Autodesk Inventor part; units mm, degrees
ref_plane "YZ Plane" through (0, 0, 0) normal (1, 0, 0) x (0, 1, 0)
ref_plane "XZ Plane" through (0, 0, 0) normal (0, 1, 0) x (-1, 0, 0)
ref_plane "XY Plane" through (0, 0, 0) normal (0, 0, 1) x (1, 0, 0)
sketch "Sketch1" plane through (0, 0, 0) normal (0, 0, 1) x (1, 0, 0)
  circle A0 centre (0, 0) radius 55
  arc A1 (-1.4, -192.7776) -> (1.4, -192.7776) centre (0, -192.7776) ccw
  line L0 (-95, 160) -> (105, 160)
  line L1 (105, 160) -> (105, -240)
  line L2 (105, -240) -> (-95, -240)
  line L3 (-95, -240) -> (-95, 160)
  line L4 (-95, 200) -> (95, -200) construction
  line L5 (95, 200) -> (-95, -200) construction
  line L6 (0, 0) -> (0, -40) construction
  point P0 (0, 0)
  dimension "d58" = 200
  dimension "d59" = 400
  dimension "d60" = 40
extrude "Extrusion1" add sketch "Sketch1" against normal blind 5
sketch "Sketch2" plane through (0, 0, 0) normal (0, 0, 1) x (1, 0, 0)
  circle A0 centre (-22.5, -100.6741) radius 2.25
  circle A1 centre (22.5, -100.6741) radius 2.25
  circle A2 centre (22.5, -71.1776) radius 2
  circle A3 centre (-22.5, -71.1776) radius 2
  circle A4 centre (-22.5, -162.7577) radius 2.25
  circle A5 centre (22.5, -162.7577) radius 2.25
  point P0 (0, 0)
  dimension "d53" = 71.1776
  dimension "d54" = 100.6741
  dimension "d55" = 162.7577
hole "Hole1" at (22.5, -71.1776, 0) at (-22.5, -71.1776, 0) at (-22.5, -100.6741, 0) at (22.5, -100.6741, 0) at (-22.5, -162.7577, 0) at (22.5, -162.7577, 0) direction (0, 0, -1) diameter 4 end through all
sketch "Sketch3" plane through (0, 0, 0) normal (0, 0, 1) x (1, 0, 0)
  line L0 (1.9053, 65.8) -> (3.8105, 62.5)
  line L1 (-1.9053, 65.8) -> (1.9053, 65.8)
  line L2 (-3.8105, 62.5) -> (-1.9053, 65.8)
  line L3 (-1.9053, 59.2) -> (-3.8105, 62.5)
  line L4 (1.9053, 59.2) -> (-1.9053, 59.2)
  line L5 (3.8105, 62.5) -> (1.9053, 59.2)
  line L6 (-33.2555, 49.0137) -> (-36.3383, 46.7739)
  line L7 (-33.6538, 52.8033) -> (-33.2555, 49.0137)
  line L8 (-37.1349, 54.3532) -> (-33.6538, 52.8033)
  line L9 (-40.2177, 52.1134) -> (-37.1349, 54.3532)
  line L10 (-39.8193, 48.3238) -> (-40.2177, 52.1134)
  line L11 (-36.3383, 46.7739) -> (-39.8193, 48.3238)
  line L12 (-55.7138, 20.1058) -> (-56.8913, 16.4818)
  line L13 (-58.2635, 22.9376) -> (-55.7138, 20.1058)
  line L14 (-61.9908, 22.1453) -> (-58.2635, 22.9376)
  line L15 (-63.1683, 18.5213) -> (-61.9908, 22.1453)
  line L16 (-60.6185, 15.6896) -> (-63.1683, 18.5213)
  line L17 (-56.8913, 16.4818) -> (-60.6185, 15.6896)
  line L18 (-56.8913, -16.4818) -> (-55.7138, -20.1058)
  line L19 (-60.6185, -15.6896) -> (-56.8913, -16.4818)
  line L20 (-63.1683, -18.5213) -> (-60.6185, -15.6896)
  line L21 (-61.9908, -22.1453) -> (-63.1683, -18.5213)
  line L22 (-58.2635, -22.9376) -> (-61.9908, -22.1453)
  line L23 (-55.7138, -20.1058) -> (-58.2635, -22.9376)
  line L24 (-36.3383, -46.7739) -> (-33.2555, -49.0137)
  line L25 (-39.8193, -48.3238) -> (-36.3383, -46.7739)
  line L26 (-40.2177, -52.1134) -> (-39.8193, -48.3238)
  line L27 (-37.1349, -54.3532) -> (-40.2177, -52.1134)
  line L28 (-33.6538, -52.8033) -> (-37.1349, -54.3532)
  line L29 (-33.2555, -49.0137) -> (-33.6538, -52.8033)
  line L30 (33.2555, -49.0137) -> (36.3383, -46.7739)
  line L31 (33.6538, -52.8033) -> (33.2555, -49.0137)
  line L32 (37.1349, -54.3532) -> (33.6538, -52.8033)
  line L33 (40.2177, -52.1134) -> (37.1349, -54.3532)
  line L34 (39.8193, -48.3238) -> (40.2177, -52.1134)
  line L35 (36.3383, -46.7739) -> (39.8193, -48.3238)
  line L36 (55.7138, -20.1058) -> (56.8913, -16.4818)
  line L37 (58.2635, -22.9376) -> (55.7138, -20.1058)
  line L38 (61.9908, -22.1453) -> (58.2635, -22.9376)
  line L39 (63.1683, -18.5213) -> (61.9908, -22.1453)
  line L40 (60.6185, -15.6896) -> (63.1683, -18.5213)
  line L41 (56.8913, -16.4818) -> (60.6185, -15.6896)
  line L42 (56.8913, 16.4818) -> (55.7138, 20.1058)
  line L43 (60.6185, 15.6896) -> (56.8913, 16.4818)
  line L44 (63.1683, 18.5213) -> (60.6185, 15.6896)
  line L45 (61.9908, 22.1453) -> (63.1683, 18.5213)
  line L46 (58.2635, 22.9376) -> (61.9908, 22.1453)
  line L47 (55.7138, 20.1058) -> (58.2635, 22.9376)
  line L48 (36.3383, 46.7739) -> (33.2555, 49.0137)
  line L49 (39.8193, 48.3238) -> (36.3383, 46.7739)
  line L50 (40.2177, 52.1134) -> (39.8193, 48.3238)
  line L51 (37.1349, 54.3532) -> (40.2177, 52.1134)
  line L52 (33.6538, 52.8033) -> (37.1349, 54.3532)
  line L53 (33.2555, 49.0137) -> (33.6538, 52.8033)
  circle A0 centre (0, 0) radius 42
  line L54 (1.9053, 65.8) -> (-1.9053, 59.2)
  line L55 (-3.8105, 62.5) -> (3.8105, 62.5)
  arc A1 (41.8018, -53.634) -> (-41.8018, -53.634) centre (0, 0) ccw
  arc A2 (31.3377, -53) -> (41.8018, -53.634) centre (36.7366, -50.5636) ccw
  line L56 (-31.3377, -53) -> (31.3377, -53)
  arc A3 (-41.8018, -53.634) -> (-31.3377, -53) centre (-36.7366, -50.5636) ccw
  point P0 (0, 0)
  point P1 (0, 62.5)
  point P2 (-36.7366, 50.5636)
  point P3 (0, 0)
  point P4 (-59.441, 19.3136)
  point P5 (0, 0)
  point P6 (-59.441, -19.3136)
  point P7 (0, 0)
  point P8 (-36.7366, -50.5636)
  point P9 (0, 0)
  point P10 (0, -62.5)
  point P11 (0, 0)
  point P12 (36.7366, -50.5636)
  point P13 (0, 0)
  point P14 (59.441, -19.3136)
  point P15 (0, 0)
  point P16 (59.441, 19.3136)
  point P17 (0, 0)
  point P18 (36.7366, 50.5636)
  point P19 (0, 0)
hole "Hole2" at (0, 62.5, 0) at (-36.7366, 50.5636, 0) at (-59.441, 19.3136, 0) at (-59.441, -19.3136, 0) at (-36.7366, -50.5636, 0) at (0, -62.5, 0) at (36.7366, -50.5636, 0) at (59.441, -19.3136, 0) at (59.441, 19.3136, 0) at (36.7366, 50.5636, 0) direction (0, 0, -1) diameter 4 end through all
sketch "Sketch4" plane through (0, 0, 0) normal (0, 0, 1) x (1, 0, 0)
  circle A0 centre (-2.7145, -65.4202) radius 7.4729
  point P0 (0, 0)
extrude "Extrusion2" add sketch "Sketch4" against normal blind 5
sketch "Sketch6" plane through (0, 0, 0) normal (0, 0, 1) x (1, 0, 0)
  circle A0 centre (0, 0) radius 27.5
  circle A1 centre (59.441, 19.3136) radius 2
  circle A2 centre (36.7366, -50.5636) radius 2
  circle A3 centre (-36.7366, -50.5636) radius 2
  circle A4 centre (-59.441, 19.3136) radius 2
  circle A5 centre (0, 62.5) radius 2
  circle A6 centre (-36.7366, 50.5636) radius 2
  circle A7 centre (-59.441, -19.3136) radius 2
  circle A8 centre (59.441, -19.3136) radius 2
  circle A9 centre (36.7366, 50.5636) radius 2
  circle A10 centre (-22.5, -162.7577) radius 2
  circle A11 centre (-22.5, -100.6741) radius 2
  circle A12 centre (22.5, -71.1776) radius 2
  circle A13 centre (-22.5, -71.1776) radius 2
  circle A14 centre (22.5, -100.6741) radius 2
  circle A15 centre (22.5, -162.7577) radius 2
  circle A16 centre (0, 0) radius 55
  dimension "d38" = 55
extrude "Extrusion3" add sketch "Sketch6" against normal up to surface (5 mm away) contours A16
sketch "Sketch9" plane through (0, 0, 0) normal (0, 0, 1) x (1, 0, 0)
  circle A0 centre (0, 0) radius 27.5
  circle A1 centre (59.441, 19.3136) radius 2
  circle A2 centre (36.7366, -50.5636) radius 2
  circle A3 centre (-36.7366, -50.5636) radius 2
  circle A4 centre (-59.441, 19.3136) radius 2
  circle A5 centre (0, 62.5) radius 2
  circle A6 centre (-36.7366, 50.5636) radius 2
  circle A7 centre (-59.441, -19.3136) radius 2
  circle A8 centre (59.441, -19.3136) radius 2
  circle A9 centre (36.7366, 50.5636) radius 2
  circle A10 centre (-22.5, -162.7577) radius 2
  circle A11 centre (-22.5, -100.6741) radius 2
  circle A12 centre (22.5, -71.1776) radius 2
  circle A13 centre (-22.5, -71.1776) radius 2
  circle A14 centre (22.5, -100.6741) radius 2
  circle A15 centre (22.5, -162.7577) radius 2
  line L0 (-95, -240) -> (105, -240)
  line L1 (105, -240) -> (105, 160)
  line L2 (105, 160) -> (-95, 160)
  line L3 (-95, 160) -> (-95, -240)
  line L4 (-85, -230) -> (95, -230) construction
  line L5 (95, -230) -> (95, 150) construction
  line L6 (95, 150) -> (-85, 150) construction
  line L7 (-85, 150) -> (-85, -230) construction
  line L8 (-95, -240) -> (-95, 160) construction
  line L9 (-95, -230) -> (-75, -230) construction
  point P0 (-35, -230)
  point P1 (5, -230)
  point P2 (45, -230)
  point P3 (85, -230)
  point P4 (-75, 150)
  point P5 (-35, 150)
  point P6 (5, 150)
  point P7 (45, 150)
  point P8 (85, 150)
  dimension "d61" = 10
  dimension "d62" = 20
  dimension "d65" = 40
  dimension "d68" = 380
hole "Hole4" at (-75, -230, 0) at (-35, -230, 0) at (5, -230, 0) at (45, -230, 0) at (85, -230, 0) at (-75, 150, 0) at (-35, 150, 0) at (5, 150, 0) at (45, 150, 0) at (85, 150, 0) direction (0, 0, -1) diameter 6 end through all
sketch "Sketch10" plane through (0, 0, 0) normal (0, 0, 1) x (1, 0, 0)
  circle A0 centre (45, 150) radius 3
  circle A1 centre (-35, 150) radius 3
  circle A2 centre (85, -230) radius 3
  circle A3 centre (5, -230) radius 3
  circle A4 centre (-75, -230) radius 3
  circle A5 centre (-35, -230) radius 3
  circle A6 centre (45, -230) radius 3
  circle A7 centre (-75, 150) radius 3
  circle A8 centre (5, 150) radius 3
  circle A9 centre (85, 150) radius 3
  circle A10 centre (0, 0) radius 27.5
  circle A11 centre (59.441, 19.3136) radius 2
  circle A12 centre (36.7366, -50.5636) radius 2
  circle A13 centre (-36.7366, -50.5636) radius 2
  circle A14 centre (-59.441, 19.3136) radius 2
  circle A15 centre (0, 62.5) radius 2
  circle A16 centre (-36.7366, 50.5636) radius 2
  circle A17 centre (-59.441, -19.3136) radius 2
  circle A18 centre (59.441, -19.3136) radius 2
  circle A19 centre (36.7366, 50.5636) radius 2
  circle A20 centre (-22.5, -162.7577) radius 2
  circle A21 centre (-22.5, -100.6741) radius 2
  circle A22 centre (22.5, -71.1776) radius 2
  circle A23 centre (-22.5, -71.1776) radius 2
  circle A24 centre (22.5, -100.6741) radius 2
  circle A25 centre (22.5, -162.7577) radius 2
  line L0 (-95, -240) -> (105, -240)
  line L1 (105, -240) -> (105, 160)
  line L2 (105, 160) -> (-95, 160)
  line L3 (-95, 160) -> (-95, -240)
  line L4 (-85, -230) -> (95, -230)
  line L5 (95, -230) -> (95, 150)
  line L6 (95, 150) -> (-85, 150)
  line L7 (-85, 150) -> (-85, -230)
  line L8 (-85, -230) -> (-85, -200)
  point P0 (-85, -160)
  point P1 (-85, -120)
  point P2 (-85, -80)
  point P3 (-85, -40)
  point P4 (-85, 0)
  point P5 (-85, 40)
  point P6 (-85, 80)
  point P7 (-85, 120)
  point P8 (95, -200)
  point P9 (95, -160)
  point P10 (95, -120)
  point P11 (95, -80)
  point P12 (95, -40)
  point P13 (95, 0)
  point P14 (95, 40)
  point P15 (95, 80)
  point P16 (95, 120)
  dimension "d78" = 10
  dimension "d79" = 30
  dimension "d82" = 40
  dimension "d85" = 180
hole "Hole5" at (-85, -200, 0) at (-85, -160, 0) at (-85, -120, 0) at (-85, -80, 0) at (-85, -40, 0) at (-85, 0, 0) at (-85, 40, 0) at (-85, 80, 0) at (-85, 120, 0) at (95, -200, 0) at (95, -160, 0) at (95, -120, 0) at (95, -80, 0) at (95, -40, 0) at (95, 0, 0) at (95, 40, 0) at (95, 80, 0) at (95, 120, 0) direction (0, 0, -1) diameter 6 end through all
properties part number "Podstawa" material "Aluminum 6061"
Geometry: final body of the model. Coordinates: model frame, mm. Round coordinates to 2 decimals unless told otherwise and drop trailing zeros. Loops run counter-clockwise (first coordinate to the right, second up) from the corner with the lowest first, then second, coordinate; pieces in that order, holes last.
Q1. Section B-B on z = -4. State how many separate pieces and enclosed holes the cut face has, plus the area to 3 significant figures.
Q2. Section A-A on x = 14.5. Return loops of the section in (y, z), plus the area to 3 significant figures.
Q3. Pull-direction query (X, two-part tool) for faces 1 (the flat face through (4, -37, -5)), 2 (the cylindrical face through (-5.961, -26.846, -2.465)); classes: released by +X, released by -X, zero draft, split by the parting line, or undercut.
Q4. Material intervals for L1, parallel to X at y = 40, z = -1.5; L2, parallel to Y at x = -34, z = -1.5; L3, parallel to X at y = -202.5, z = -0.2, sorted ascending.
Q5. Pin query (flat end, axial travel): P1, Ø4.5, axis at x = -59.44, y = 19.31, coming from the -Z side. Return the tip coordinate at first contact, or that it passes through.
Evaluation:
1. separate pieces: 1
1. enclosed holes: 44
1. area: 76,600 mm2
2. outline: (-240, -5) - (-23.37, -5) - (-23.37, 0) - (-240, 0) - close; (23.37, -5) - (160, -5) - (160, 0) - (23.37, 0) - close
2. area: 1,770 mm2
3. face 1: zero draft
3. face 2: undercut
4. L1: x = -95 to -88, -82 to 92, 98 to 105
4. L2: y = -240 to -232.83, -227.17 to 147.17, 152.83 to 160
4. L3: x = -95 to -86.66, -83.34 to 93.34, 96.66 to 105
5. P1: stops at z = -5
